from build123d import *

# Parameters (mm, degrees)
SKETCH1_R               = 57.75
BOSS_EXTRUDE2_DEPTH     = 12
BOSS_EXTRUDE3_DEPTH     = 21
SKETCH2_W               = 101
SKETCH2_H               = 51
CUT_EXTRUDE1_DEPTH      = 5
SKETCH4_W               = 21
SKETCH4_H               = 20
CUT_EXTRUDE2_DEPTH      = 8
SKETCH5_W               = 21
SKETCH5_H               = 40.810106116
CUT_EXTRUDE3_DEPTH      = 35
CUT_EXTRUDE3_DEPTH_BACK = 3
SKETCH6_W               = 21
SKETCH6_H               = 10.991891623
BOSS_EXTRUDE4_DEPTH     = 3
SKETCH9_R               = 2
CUT_EXTRUDE6_DEPTH      = 31
SKETCH12_R              = 9.75
BOSS_EXTRUDE5_DEPTH     = 9
SKETCH7_R               = 1.4
BOSS_EXTRUDE6_DEPTH     = 7
SKETCH7_6_R             = 1.5
CUT_EXTRUDE10_DEPTH     = 10
CHAMFER1_SIZE           = 10


with BuildPart() as part:
    # Sketch1 → Boss-Extrude2 (new body)
    with BuildSketch(Plane.XY):
        with Locations((-3.428783881, -2.741891623)):
            Circle(SKETCH1_R)
    extrude(amount=BOSS_EXTRUDE2_DEPTH)

    # Sketch1<4> → Boss-Extrude3 (add)
    with BuildSketch(Plane.XY):
        with BuildLine():
            Line((-54.304676832, 48.558264482), (-44.094290011, 38.262731423))
            ThreePointArc((-44.094290011, 38.262731423), (-3.428783881, 55.008108377), (37.23672225, 38.262731423))
            Line((37.23672225, 38.262731423), (47.44710907, 48.558264482))
            ThreePointArc((47.44710907, 48.558264482), (-3.428783881, 69.508108377), (-54.304676832, 48.558264482))
        make_face()
        with BuildLine():
            ThreePointArc((37.23672225, -43.746514669), (-3.428783881, -60.491891623), (-44.094290011, -43.746514669))
            Line((-44.094290011, -43.746514669), (-54.304676832, -54.042047728))
            ThreePointArc((-54.304676832, -54.042047728), (-3.428783881, -74.991891623), (47.44710907, -54.042047728))
            Line((47.44710907, -54.042047728), (37.23672225, -43.746514669))
        make_face()
    extrude(amount=BOSS_EXTRUDE3_DEPTH)

    # Sketch2 → Cut-Extrude1 (cut)
    with BuildSketch(Plane(origin=(0, 0, 0), x_dir=(-1, 0, 0), z_dir=(0, 0, -1))):
        with Locations((3.428783881, -2.741891623)):
            Rectangle(SKETCH2_W, SKETCH2_H)
    extrude(amount=-CUT_EXTRUDE1_DEPTH, mode=Mode.SUBTRACT)

    # Sketch4 → Cut-Extrude2 (cut)
    with BuildSketch(Plane(origin=(0, 0, 5), x_dir=(-1, 0, 0), z_dir=(0, 0, -1))):
        with Locations((3.428783881, -0.991891623)):
            Rectangle(SKETCH4_W, SKETCH4_H)
    extrude(amount=-CUT_EXTRUDE2_DEPTH, mode=Mode.SUBTRACT)

    # Sketch5 → Cut-Extrude3 (cut, two sides)
    with BuildSketch(Plane(origin=(0, 0, 5), x_dir=(-1, 0, 0), z_dir=(0, 0, -1))) as cut_extrude3_sk:
        with Locations((3.428783881, 9.413161435)):
            Rectangle(SKETCH5_W, SKETCH5_H)
    extrude(amount=CUT_EXTRUDE3_DEPTH, mode=Mode.SUBTRACT)
    extrude(cut_extrude3_sk.sketch, amount=-CUT_EXTRUDE3_DEPTH_BACK, mode=Mode.SUBTRACT)

    # Sketch6 → Boss-Extrude4 (add)
    with BuildSketch(Plane(origin=(0, 0, 5), x_dir=(-1, 0, 0), z_dir=(0, 0, -1))):
        with Locations((3.428783881, -5.495945812)):
            Rectangle(SKETCH6_W, SKETCH6_H)
    extrude(amount=-BOSS_EXTRUDE4_DEPTH)

    # Sketch9 → Cut-Extrude6 (cut)
    with BuildSketch(Plane.XY.offset(12)):
        with Locations((-45.928783881, -17.741891623)):
            Circle(SKETCH9_R)
        with Locations((-45.928783881, 12.258108377)):
            Circle(SKETCH9_R)
        with Locations((39.071216119, 12.258108377)):
            Circle(SKETCH9_R)
        with Locations((39.071216119, -17.741891623)):
            Circle(SKETCH9_R)
    extrude(amount=-CUT_EXTRUDE6_DEPTH, mode=Mode.SUBTRACT)

    # Sketch12 → Boss-Extrude5 (add)
    with BuildSketch(Plane.XY.offset(12)):
        with Locations((-3.428783881, -44.741891623)):
            Circle(SKETCH12_R)
        with Locations((-3.428783881, 39.258108377)):
            Circle(SKETCH12_R)
    extrude(amount=BOSS_EXTRUDE5_DEPTH)

    # Sketch7 → Boss-Extrude6 (add)
    with BuildSketch(Plane(origin=(0, 0, 5), x_dir=(-1, 0, 0), z_dir=(0, 0, -1))):
        with Locations((10.928783881, -7.241891623)):
            Circle(SKETCH7_R)
    extrude(amount=-BOSS_EXTRUDE6_DEPTH)

    # Sketch7<6> → Cut-Extrude10 (cut)
    with BuildSketch(Plane(origin=(0, 0, 5), x_dir=(-1, 0, 0), z_dir=(0, 0, -1))):
        with Locations((-4.071216119, -7.241891623)):
            Circle(SKETCH7_6_R)
    extrude(amount=-CUT_EXTRUDE10_DEPTH, mode=Mode.SUBTRACT)

    # Chamfer1
    chamfer1_edges = [part.edges().sort_by_distance(p)[0] for p in [
        (-3.428783881, -74.991891623, 0),
        (-3.428783881, 69.508108377, 0),
    ]]
    chamfer(chamfer1_edges, length=CHAMFER1_SIZE)


solid = part.part
The listing builds one solid part. Answer for the finished solid, in the listing's coordinates (mm). A direction names the side the tool comes from. Round coordinates to 2 decimals unless told otherwise and drop trailing zeros. Loops run counter-clockwise (first coordinate to the right, second up) from the corner with the lowest first, then second, coordinate; pieces in that order, holes last. Notation, with made-up numbers: M 1,-25.75 L 55,-25.75 A22 cw 55,-19.75 Z; hole C 65,-12.5 d8. An arc over 180 degrees is marked long. Return JSON: item names as keys, results as strings.
Q1. Which of the six approach directions +Z, -Z, +X, -X, +Y, -Y give full straight-line access (tool end or side, diameter ignored) to faces 1 (the face through (47.071, -3, 2)), 2 (the face through (9, -2, 12)), 3 (the face through (-4.219, -74.988, 15.423)), 4 (the face through (-13.929, 9, 7)), 5 (the face through (-3, 0, 6))?
Results list:
{"face 1": "-Z", "face 2": "+Z", "face 3": "+Z, -Z, -Y", "face 4": "none", "face 5": "+Z, -Z"}
Q2. Find section B-B, the plane y = -40. Determine the outline of the cut face in (x, z).
Results list:
{"outline": "M -47.55,0 L 40.69,0 L 40.69,12 L 5.09,12 L 5.09,21 L -11.95,21 L -11.95,12 L -47.55,12 Z"}
Q3. Find section C-C, the plane z = 1.5. Determine the outline of the cut face in (x, y), plus the area to 3 significant figures.
Results list:
{"outline": "M -48.32,-48.01 A63.75 ccw 41.46,-48.01 L 37.24,-43.75 A57.75 ccw 37.24,38.26 L 41.46,42.52 A63.75 ccw -48.32,42.52 L -44.09,38.26 A57.75 ccw -44.09,-43.75 Z; hole M -53.93,-28.24 L 47.07,-28.24 L 47.07,22.76 L 7.07,22.76 L 7.07,29.82 L -13.93,29.82 L -13.93,22.76 L -53.93,22.76 Z", "area": "6,320 mm2"}
Q4. The mould has two halves that part along X. Classify faces 6 (the face through (7.071, 9, 7)), 7 (the face through (-4, -63, 21)), 8 (the face through (-53.929, -3, 2)), 9 (the face through (-2.729, 61.241, 1.737)): released by +X, released by -X, zero draft, split by the parting line, or undercut.
Results list:
{"face 6": "undercut", "face 7": "zero draft", "face 8": "undercut", "face 9": "split by the parting line"}
Q5. Find section D-D, the plane y = -4. Determine the outline of the cut face in (x, z).
Results list:
{"outline": "M -61.17,0 L -53.93,0 L -53.93,5 L 47.07,5 L 47.07,0 L 54.31,0 L 54.31,12 L 7.07,12 L 7.07,8 L -13.93,8 L -13.93,12 L -61.17,12 Z"}
Q6. Each of these flat-tipped pins is pushed along its axis until it touches: pin 1 Ø3.5 at (x, z) = (-6.5, 6) entering from +Y; pin 2 Ø3 at (x, y) = (-46.5, -32) entering from +Z; pin 3 Ø5 at (y, z) = (52, 16) entering from -X; pin 4 Ø2.5 at (x, y) = (4.07, -7.24) entering from -Z (1 decimal). Where does it stop, or does it pass through?
Results list:
{"pin 1": "stops at y = 67.19", "pin 2": "stops at z = 12", "pin 3": "stops at x = -53.34", "pin 4": "passes through"}
Q7. Find section A-A, the plane z = 13.75. Determine the outline of the cut face in (x, y), plus the area to 3 significant figures.
Results list:
{"outline": "M -54.3,-54.04 A72.25 ccw 47.45,-54.04 L 37.24,-43.75 A57.75 cw -44.09,-43.75 Z; M -54.3,48.56 L -44.09,38.26 A57.75 cw 37.24,38.26 L 47.45,48.56 A72.25 ccw Z; C -3.43,-44.74 d19.5; C -3.43,39.26 d19.5", "area": "3,540 mm2"}
Q8. Find the intervals of material crossed by line 1 along X through (y, z) = (42.5, 13.5); line 2 along X through (y, z) = (10.5, 9.25); line 3 along Z through (x, y) = (-37, 1.5), in increasing order. Write a range as from..to.
Results list:
{"line 1": "x = -48.3..-39.32, -12.62..5.77, 32.46..41.44", "line 2": "x = -59.64..-46.88, -44.98..38.12, 40.02..52.78", "line 3": "z = 5..12"}
